Check sheet for the modelled part. Datum: model origin and axes. Units: mm. A direction names the side the tool comes from. Round coordinates to 2 decimals unless told otherwise and drop trailing zeros. Loops run counter-clockwise (first coordinate to the right, second up) from the corner with the lowest first, then second, coordinate; pieces in that order, holes last. Notation, with made-up numbers: (-13, -21.5) -> (4, -21.5) arc R20 cw to (4, -17.5) -> close; hole circle Ø4 at (24, -2.5). An arc over 180 degrees is marked (long way). Return JSON: item names as keys, results as strings.
from build123d import *

# Parameters (mm, degrees)
SKETCH1_W           = 50.8
SKETCH1_H           = 50.8
BOSS_EXTRUDE1_DEPTH = 3
SKETCH2_W           = 3
SKETCH2_H           = 7.16
SKETCH2_W_2         = 10.16
SKETCH2_H_2         = 3
SKETCH2_H_3         = 10.16
CUT_EXTRUDE1_DEPTH  = 72.904659098


with BuildPart() as part:
    # Sketch1 → Boss-Extrude1 (new body)
    with BuildSketch(Plane(origin=(0, 0, 0), x_dir=(1, 0, 0), z_dir=(0, 1, 0))):
        with Locations((25.4, 25.4)):
            Rectangle(SKETCH1_W, SKETCH1_H)
    extrude(amount=BOSS_EXTRUDE1_DEPTH)

    # Sketch2 → Cut-Extrude1 (cut, through all)
    with BuildSketch(Plane(origin=(0, 3, 0), x_dir=(1, 0, 0), z_dir=(0, 1, 0))):
        with Locations((1.5, 44.22)):
            Rectangle(SKETCH2_W, SKETCH2_H)
        Polygon((10.16, 47.8), (10.16, 50.8), (0, 50.8), (0, 47.8), (3, 47.8), align=None)
        with Locations((25.4, 49.3)):
            Rectangle(SKETCH2_W_2, SKETCH2_H_2)
        Polygon((50.8, 50.8), (40.64, 50.8), (40.64, 47.8), (47.8, 47.8), (50.8, 47.8), align=None)
        with Locations((49.3, 44.22)):
            Rectangle(SKETCH2_W, SKETCH2_H)
        with Locations((49.3, 25.4)):
            Rectangle(SKETCH2_W, SKETCH2_H_3)
        with Locations((49.3, 6.58)):
            Rectangle(SKETCH2_W, SKETCH2_H)
        Polygon((50.8, 0), (50.8, 3), (47.8, 3), (40.64, 3), (40.64, 0), align=None)
        with Locations((25.4, 1.5)):
            Rectangle(SKETCH2_W_2, SKETCH2_H_2)
        Polygon((3, 3), (0, 3), (0, 0), (10.16, 0), (10.16, 3), align=None)
        with Locations((1.5, 6.58)):
            Rectangle(SKETCH2_W, SKETCH2_H)
        with Locations((1.5, 25.4)):
            Rectangle(SKETCH2_W, SKETCH2_H_3)
    extrude(amount=-CUT_EXTRUDE1_DEPTH, mode=Mode.SUBTRACT)


solid = part.part
Q1. Tool access check on faces 5 (the flat face through (49, 2, -40.64)), 6 (the flat face through (47.8, 2, -25)), 7 (the flat face through (25, 2, -3)). Record the directions out of +Z, -Z, +X, -X, +Y, -Y that give a thin tool (end or side, any length) a straight path to the whole face; none if there is none.
Results list:
{"face 5": "-Z, +X, +Y, -Y", "face 6": "+X, +Y, -Y", "face 7": "+Z, +Y, -Y"}
Q2. Material ranges on line 1 (X direction, y = 2.45, z = -22); line 2 (X direction, y = 2.7, z = -2); line 3 (Z direction, x = 48, y = 2.75), recorded low to high.
Results list:
{"line 1": "3 to 47.8", "line 2": "10.16 to 20.32, 30.48 to 40.64", "line 3": "-40.64 to -30.48, -20.32 to -10.16"}
Q3. Go/stop test with flat-tipped pins: pin 1 (12 mm diameter, centred on x = 15.5, z = -7, fed in from -Y); pin 2 (1.5 mm diameter, centred on y = 1.5, z = -8, fed in from +X); pin 3 (1.5 mm diameter, centred on x = 6, y = 1.5, fed in from +Z); pin 4 (1.5 mm diameter, centred on y = 1.5, z = -24, fed in from -X). Record where each tip stops, or that it passes through.
Results list:
{"pin 1": "y = 0", "pin 2": "x = 47.8", "pin 3": "z = -3", "pin 4": "x = 3"}
Q4. Draft check along X on faces 1 (the flat face through (20.32, 2, -1)), 2 (the flat face through (35, 1, 0)), 3 (the flat face through (3, 2, -44)), 4 (the flat face through (30.48, 2, -49)). Enter one of: released by +X, released by -X, zero draft, split by the parting line, or undercut.
Results list:
{"face 1": "undercut", "face 2": "zero draft", "face 3": "released by -X", "face 4": "undercut"}
Q5. Section check A-A (z = -44). Record the boundary of the cut face in (x, y), then the cut area to 3 significant figures.
Results list:
{"outline": "(3, 0) -> (47.8, 0) -> (47.8, 3) -> (3, 3) -> close", "area": "134 mm^2"}
